For this review, take the finished solid that the model builds, in its own axes (mm). A direction names the side the tool comes from. Coordinates: 2 decimals unless noted, no trailing zeros. Order: outer loops, then holes, each group sorted by start corner. A loop starts at its lowest first (then second) coordinate and runs counter-clockwise, first axis right, second up. Notation, with made-up numbers: M -34,0.5 L 21,0.5 A24 ccw 21,38.5 Z; hole C 48,6 d8. An arc over 180 degrees is marked long. Use one line per item in the form item = value. Start each with the question number.
```python
from build123d import *

# Parameters (mm, degrees)
SKETCH1_W                  = 0.636
SKETCH1_H                  = 0.636
BOSS_EXTRUDE1_DEPTH        = 2.54
BOSS_EXTRU_1_DEPTH         = 0.64
R_P_TITION_LIN_AIRE1_COUNT = 10
R_P_TITION_LIN_AIRE1_PITCH = 2.54


with BuildPart() as part:
    # Sketch1 → Boss-Extrude1 (new body)
    with BuildSketch(Plane.XZ):
        Polygon((-0.353553391, -2.186446609), (-2.186446609, -2.186446609), (-2.54, -1.832893219), (-2.54, 0), (-2.186446609, 0.353553391), (-0.353553391, 0.353553391), (0, 0), (0, -1.832893219), align=None)
        with Locations((-1.27, -0.916446609)):
            Rectangle(SKETCH1_W, SKETCH1_H, mode=Mode.SUBTRACT)
    boss_extrude1 = extrude(amount=-BOSS_EXTRUDE1_DEPTH)

    # Esquisse1 → Boss.-Extru.1 (add)
    with BuildSketch(Plane(origin=(-1.588, 0, 0), x_dir=(0, 0, -1), z_dir=(1, 0, 0))):
        with BuildLine():
            Line((0.598446609, 8.54), (0.598446609, -0.18))
            ThreePointArc((0.598446609, -0.18), (1.037786438, -1.240660172), (2.098446609, -1.68))
            Line((2.098446609, -1.68), (5.488446609, -1.68))
            Line((5.488446609, -1.68), (5.488446609, -1.04))
            Line((5.488446609, -1.04), (2.098446609, -1.04))
            ThreePointArc((2.098446609, -1.04), (1.490334778, -0.788111832), (1.238446609, -0.18))
            Line((1.238446609, -0.18), (1.238446609, 8.54))
            Line((1.238446609, 8.54), (0.598446609, 8.54))
        make_face()
    boss_extru_1 = extrude(amount=BOSS_EXTRU_1_DEPTH)

    # Répétition linéaire1: Boss-Extrude1, Boss.-Extru.1 ×10
    with Locations(*[(i * R_P_TITION_LIN_AIRE1_PITCH, 0, 0) for i in range(1, R_P_TITION_LIN_AIRE1_COUNT)]):
        add(boss_extrude1)
        add(boss_extru_1)


solid = part.part
```
1. For pin 1 Ø2 at (y, z) = (7.5, -1) entering from -X; pin 2 Ø0.5 at (x, y) = (6.5, 6) entering from +Z; pin 3 Ø6 at (x, y) = (4.5, 5) entering from -Z, all flat-tipped, find the tip position at first contact; note any pin that passes through.
2. Tool access review of faces 4 (the flat face through (14.292, -1.2, -3)), 5 (the cylindrical face through (6.3, -0.8, -1.5)), 6 (the cylindrical face through (21.6, -1.2, -1)), 7 (the flat face through (9, 1, -2.186)): name each direction out of +Z, -Z, +X, -X, +Y, -Y from which nothing blocks a thin tool from reaching the whole face with its end or side.
3. The part is to be moulded in two halves that separate along Y. For faces 1 (the cylindrical face through (8.9, -1.2, -1)), 2 (the cylindrical face through (1.3, -0.8, -1.5)), 3 (the flat face through (22, 1, -2.186)), say which applies: pulls with the +Y half, pulls with the -Y half, needs draft (parallel to the pull), parting line crosses it, or undercut.
4. To check wall thickness, follow line 1 (Y direction, x = 4.25, z = -0.2); line 2 (Z direction, x = 4, y = 2.5); line 3 (Y direction, x = 16.25, z = -4.7). State the ranges of each line that lie inside material, in increasing order.
5. Consider section A-A, the plane x = 18.5. Write out the cut boundary in (y, z), plus the area to 3 significant figures.
6. Consider section D-D, the plane z = -0.3. Write out the cut boundary in (x, y), plus the area to 3 significant figures.
7. Consider section B-B, the plane z = -3.4. Give the number of separate pieces and of enclosed holes in the cut face, plus the area to 3 significant figures.
Answers follow:
q1.pin_1 = -1.59
q1.pin_2 = -0.6
q1.pin_3 = -2.19
q2.face_4 = +Z, -Z, -Y
q2.face_5 = -Z, +X, -X
q2.face_6 = +Z, +X, -X, -Y
q2.face_7 = -Z, +X, -X, +Y
q3.face_1 = pulls with the -Y half
q3.face_2 = undercut
q3.face_3 = needs draft
q4.line_1 = 0 to 2.54
q4.line_2 = -2.19 to 0.35
q4.line_3 = -1.68 to -1.04
q5.outline = M 0,-2.19 L 2.54,-2.19 L 2.54,0.35 L 0,0.35 Z
q5.area = 6.45 mm²
q6.outline = M -2.54,0 L 22.86,0 L 22.86,2.54 L -2.54,2.54 Z
q6.area = 64.5 mm²
q7.separate_pieces = 10
q7.enclosed_holes = 0
q7.area = 4.10 mm²
